Here's how the part is built. I have some questions about the finished solid (model axes, mm). A direction names the side the tool comes from. Give positions to 0.01 mm unless a question says otherwise; leave off trailing zeros. Loops run counter-clockwise (first coordinate to the right, second up) from the corner with the lowest first, then second, coordinate; pieces in that order, holes last. Notation, with made-up numbers: (19.5, 35.25) - (48.5, 35.25) arc R10 ccw to (48.5, 49.25) - close; hole circle Ø7 at (-10.5, 68.25). An arc over 180 degrees is marked (long way). One line per item, written item: value. Start each with the question number.
```python
from build123d import *

# Parameters (mm, degrees)
SKETCH2_R                = 15.494
BOSS_EXTRUDE1_DEPTH      = 57.2
SKETCH3_W                = 36
SKETCH3_H                = 27
BOSS_EXTRUDE2_DEPTH      = 58.1
BOSS_EXTRUDE3_DEPTH      = 15
BOSS_EXTRUDE3_DEPTH_BACK = 51
SKETCH4_R                = 4


with BuildPart() as part:
    # Sketch2 → Boss-Extrude1 (new body)
    with BuildSketch(Plane(origin=(0, 0, 0), x_dir=(1, 0, 0), z_dir=(0, 1, 0))):
        with Locations(Location((0, 0, 0), (0, 0, 270))):
            Circle(SKETCH2_R)
    extrude(amount=BOSS_EXTRUDE1_DEPTH)

    # Sketch3 → Boss-Extrude2 (add)
    with BuildSketch(Plane(origin=(0, 57.2, 0), x_dir=(1, 0, 0), z_dir=(0, 1, 0))):
        with Locations((9, 0)):
            Rectangle(SKETCH3_W, SKETCH3_H)
    extrude(amount=BOSS_EXTRUDE2_DEPTH)

    # Sketch4 → Boss-Extrude3 (add, two sides: drawn at the far end of the back side and taken through both)
    with BuildSketch(Plane(origin=(27, 0, 0), x_dir=(0, 0, -1), z_dir=(1, 0, 0)).offset(-BOSS_EXTRUDE3_DEPTH_BACK)):
        with Locations((0, 95.1)):
            Circle(SKETCH4_R)
    extrude(amount=BOSS_EXTRUDE3_DEPTH + BOSS_EXTRUDE3_DEPTH_BACK)


solid = part.part
```
(1) Will these pins go through, and if not, where does the flat tip stop? pin 1 (18 mm diameter, centred on x = 5.5, y = 81, fed in from -Z); pin 2 (1.6 mm diameter, centred on x = 3.5, z = -15, fed in from +Y); pin 3 (3 mm diameter, centred on y = 21, z = -12, fed in from -X); pin 4 (2 mm diameter, centred on x = -17, y = 23, fed in from +Z).
(2) If we section it at B-B on y = 95.1: List the corners of the cut face in (x, z) for me.
(3) Please list where these lines run through material, in increasing order: probe 1 along Z at (x, y) = (-9, 6.5); probe 2 along Y at (x, z) = (14.5, -9); probe 3 along Z at (x, y) = (-8, 74). Write a range as from..to.
(4) If we section it at D-D on y = 70: List the corners of the cut face in (x, z) for me, plus the area to 3 significant figures.
(5) For faces 1 (the face through (9, 86, 13.5)), 2 (the face through (9, 86, -13.5)), 3 (the face through (34.395, 99.066, 0.521)), 4 (the face through (-5.934, 28.2, 14.313)), 5 (the face through (-11, 57.2, 0)), which set-ups out of +Z, -Z, +X, -X, +Y, -Y let a thin tool reach every point of the face, with its end or its side?
(6) If we section it at C-C on z = 0: List the corners of the cut face in (x, y) for me, plus the area to 3 significant figures.
(7) If we section it at A-A on x = 0: List the corners of the cut face in (y, z) for me, plus the area to 3 significant figures.
(8) If we mould it in two halves opening along Y, with no side actions, what happens to faces 6 (the face through (9, 115.3, 0)), 7 (the face through (-9, 86, 0)), 8 (the face through (-16.605, 99.066, 0.521)), 9 (the face through (27, 86, 0))? For each: pulls with the +Y half, pulls with the -Y half, needs draft (parallel to the pull), parting line crosses it, or undercut.
Found:
1. pin 1: z = -13.5
1. pin 2: y = 57.2
1. pin 3: x = -11.39
1. pin 4: through
2. outline: (-24, -4) - (-9, -4) - (-9, -13.5) - (27, -13.5) - (27, -4) - (42, -4) - (42, 4) - (27, 4) - (27, 13.5) - (-9, 13.5) - (-9, 4) - (-24, 4) - close
3. probe 1: -12.61..12.61
3. probe 2: 57.2..115.3
3. probe 3: -13.5..13.5
4. outline: (-9, -13.5) - (27, -13.5) - (27, 13.5) - (-9, 13.5) - close
4. area: 972 mm^2
5. face 1: +Z, +X, -X, +Y
5. face 2: -Z, +X, -X, +Y
5. face 3: +X
5. face 4: -Y
5. face 5: +Z, -Z, -X
6. outline: (-24, 91.1) - (-9, 91.1) - (-9, 57.2) - (-15.49, 57.2) - (-15.49, 0) - (15.49, 0) - (15.49, 57.2) - (27, 57.2) - (27, 91.1) - (42, 91.1) - (42, 99.1) - (27, 99.1) - (27, 115.3) - (-9, 115.3) - (-9, 99.1) - (-24, 99.1) - close
6. area: 4,100 mm^2
7. outline: (0, -15.49) - (57.2, -15.49) - (57.2, -13.5) - (115.3, -13.5) - (115.3, 13.5) - (57.2, 13.5) - (57.2, 15.49) - (0, 15.49) - close
7. area: 3,340 mm^2
8. face 6: pulls with the +Y half
8. face 7: undercut
8. face 8: undercut
8. face 9: needs draft
